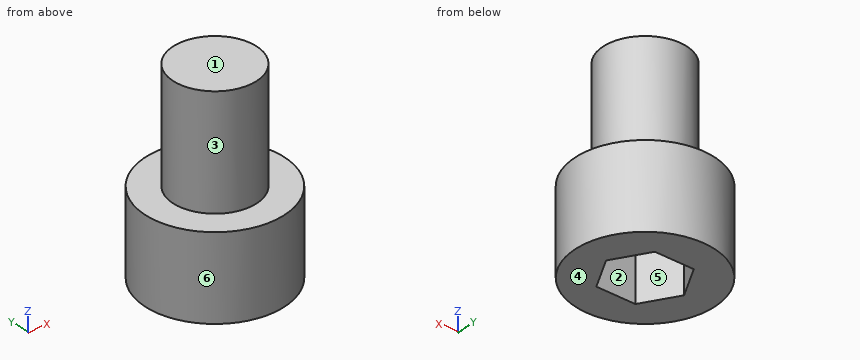
from build123d import *

# Parameters (mm, degrees)
ESBO_O1_R                = 5
RESSALTO_EXTRUS_O1_DEPTH = 6
ESBO_O2_R                = 3
RESSALTO_EXTRUS_O2_DEPTH = 8
CORTE_EXTRUS_O1_DEPTH    = 4


with BuildPart() as part:
    # Esbo_o1 → Ressalto-extrus_o1 (new body)
    # profile 1 of 2: a face of its own
    with BuildSketch(Plane.XY):
        Circle(ESBO_O1_R)
        Polygon((-1.443375673, 2.5), (-2.886751346, 0), (-1.443375673, -2.5), (1.443375673, -2.5), (2.886751346, 0), (1.443375673, 2.5), align=None, mode=Mode.SUBTRACT)
    # profile 2 of 2: a face of its own
    with BuildSketch(Plane.XY):
        Polygon((1.443375673, 2.5), (-1.443375673, 2.5), (-2.886751346, 0), (-1.443375673, -2.5), (1.443375673, -2.5), (2.886751346, 0), align=None)
    extrude(amount=RESSALTO_EXTRUS_O1_DEPTH)

    # Esbo_o2 → Ressalto-extrus_o2 (add)
    with BuildSketch(Plane.XY.offset(6)):
        Circle(ESBO_O2_R)
    extrude(amount=RESSALTO_EXTRUS_O2_DEPTH)

    # Esbo_o1_4 → Corte-extrus_o1 (cut)
    with BuildSketch(Plane.XY):
        Polygon((1.443375673, 2.5), (-1.443375673, 2.5), (-2.886751346, 0), (-1.443375673, -2.5), (1.443375673, -2.5), (2.886751346, 0), align=None)
    extrude(amount=CORTE_EXTRUS_O1_DEPTH, mode=Mode.SUBTRACT)


solid = part.part
Model file for the job. Use its own axes, mm. Face numbers are marked on the shaded views. A direction names the side the tool comes from. Round coordinates to 2 decimals unless told otherwise and drop trailing zeros. Order: outer loops, then holes, each group sorted by start corner. A loop starts at its lowest first (then second) coordinate and runs counter-clockwise, first axis right, second up.
(1) 3-axis set-ups, long thin cutter, end or side, ignore diameter. For the marked faces 1, 2 and 3: which of +Z, -Z, +X, -X, +Y, -Y reach the whole face in a straight line?
(2) Band-saw the part on D-D (z = 9). List the corners of the cut face in (x, y), then the cut area to 3 significant figures.
(3) Band-saw the part on B-B (z = 3.5). List the corners of the cut face in (x, y).
(4) Pull direction X, two halves, no side cores. Call the marked faces 4, 5 and 6: released by +X, released by -X, zero draft, split by the parting line, or undercut.
(5) Band-saw the part on A-A (x = 0). List the corners of the cut face in (y, z), then the cut area to 3 significant figures.
(6) Drill centre lines: line 1 (Z direction, x = -2.5, y = -2.75); line 2 (Z direction, x = 1.5, y = -1.75); line 3 (Y direction, x = 2.75, z = 3). Where is each one in solid material? Low to high.
(7) Band-saw the part on C-C (y = 1.75). List the corners of the cut face in (x, z), then the cut area to 3 significant figures.
(8) Pin check, flat tips, straight feed: pin 1 (2.5 mm diameter, centred on x = 0.5, z = 1.5, fed in from -Y); pin 2 (1.5 mm diameter, centred on y = 3.5, z = 7.5, fed in from +X); pin 3 (1 mm diameter, centred on x = -3.5, y = -2, fed in from +Z); pin 4 (1.5 mm diameter, centred on x = 1, y = 0.5, fed in from -Z). Stop position of each tip, or through.
Verdict:
1. face 1: +Z, +X, -X, +Y, -Y
1. face 2: -Z
1. face 3: +Z
2. outline: circle Ø6 at (0, 0)
2. area: 28.3 mm2
3. outline: circle Ø10 at (0, 0); hole (-2.89, 0) - (-1.44, -2.5) - (1.44, -2.5) - (2.89, 0) - (1.44, 2.5) - (-1.44, 2.5) - close
4. face 4: zero draft
4. face 5: undercut
4. face 6: split by the parting line
5. outline: (-5, 0) - (-2.5, 0) - (-2.5, 4) - (2.5, 4) - (2.5, 0) - (5, 0) - (5, 6) - (3, 6) - (3, 14) - (-3, 14) - (-3, 6) - (-5, 6) - close
5. area: 88.0 mm2
6. line 1: z = 0 to 6
6. line 2: z = 4 to 14
6. line 3: y = -4.18 to -0.24, 0.24 to 4.18
7. outline: (-4.68, 0) - (-1.88, 0) - (-1.88, 4) - (1.88, 4) - (1.88, 0) - (4.68, 0) - (4.68, 6) - (2.44, 6) - (2.44, 14) - (-2.44, 14) - (-2.44, 6) - (-4.68, 6) - close
7. area: 80.2 mm2
8. pin 1: stops at y = -5
8. pin 2: stops at x = 1.2
8. pin 3: stops at z = 6
8. pin 4: stops at z = 4
